from build123d import *

# Parameters (mm, degrees)
SKETCH1_W          = 120
SKETCH1_H          = 120
BASE_FLANGE1_DEPTH = 0.7366
EDGE_FLANGE1_DEPTH = 120
SKETCH25_R         = 1.5
CUT_EXTRUDE1_DEPTH = 161.891420775
CUT_EXTRUDE2_DEPTH = 10


# Sheet-metal steps are written as plain solids
with BuildPart() as part:
    # Sketch1 → Base-Flange1 (new body)
    with BuildSketch(Plane.XY):
        Rectangle(SKETCH1_W, SKETCH1_H)
    extrude(amount=-BASE_FLANGE1_DEPTH)

    # Edge-Flange1 section (across the edge) → Edge-Flange1 (add)
    with BuildSketch(Plane(origin=(-60, -61, 0), x_dir=(0, 1, 0), z_dir=(1, 0, 0))):
        with BuildLine():
            Line((-0.7366, 0.7366), (-0.7366, 24.2634))
            Line((-0.7366, 24.2634), (0, 24.2634))
            Line((0, 24.2634), (0, 0.7366))
            ThreePointArc((0, 0.7366), (0.215745145, 0.215745145), (0.7366, 0))
            Line((0.7366, 0), (1, 0))
            Line((1, 0), (1, -0.7366))
            Line((1, -0.7366), (0.7366, -0.7366))
            ThreePointArc((0.7366, -0.7366), (-0.30510971, -0.30510971), (-0.7366, 0.7366))
        make_face()
    extrude(amount=EDGE_FLANGE1_DEPTH)

    # Sketch25 → Cut-Extrude1 (cut, through all)
    with BuildSketch(Plane(origin=(-46.34767359, -57.645882303, 26.3866), x_dir=(1, 0, 0), z_dir=(0, 0, 1))):
        with Locations((-7.65232641, 6.745882303)):
            Circle(SKETCH25_R)
        with Locations((100.34767359, 113.545882303)):
            Circle(SKETCH25_R)
        with Locations((100.34767359, 6.745882303)):
            Circle(SKETCH25_R)
        with Locations((-7.65232641, 113.545882303)):
            Circle(SKETCH25_R)
    extrude(amount=-CUT_EXTRUDE1_DEPTH, mode=Mode.SUBTRACT)

    # Sketch26 → Cut-Extrude2 (cut)
    with BuildSketch(Plane(origin=(0, 0, -0.7366), x_dir=(-1, 0, 0), z_dir=(0, 0, -1))):
        Polygon((45, -15.899963077), (45, -0.320923852), (0.188671673, -45.2634), (15.722249294, -45.2634), align=None)
        Polygon((21.370855866, -45.2634), (36.904433487, -45.2634), (45, -37.144140463), (45, -21.565101238), align=None)
        Polygon((-20.993512521, -45.2634), (-5.459934899, -45.2634), (45, 5.344214309), (45, 20.923253534), align=None)
        Polygon((-45, -26.851791695), (-45, -42.43083092), (42.175696714, 45), (26.642119093, 45), align=None)
        Polygon((-45, -5.607614309), (-45, -21.186653534), (20.993512521, 45), (5.459934899, 45), align=None)
        Polygon((-45, 15.636563077), (-45, 0.057523852), (-0.188671673, 45), (-15.722249294, 45), align=None)
        Polygon((-45, 36.880740463), (-45, 21.301701238), (-21.370855866, 45), (-36.904433487, 45), align=None)
        Polygon((45, 26.588391695), (45, 42.16743092), (-42.175696714, -45.2634), (-26.642119093, -45.2634), align=None)
    extrude(amount=-CUT_EXTRUDE2_DEPTH, mode=Mode.SUBTRACT)


solid = part.part
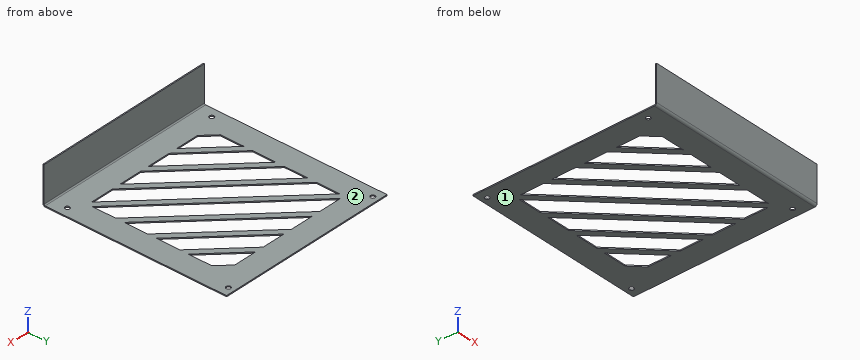
Could you check a few things on this model? Use its own coordinates, in mm. Face numbers are marked on the shaded views. A direction names the side the tool comes from. Coordinates: 2 decimals unless noted, no trailing zeros. Loops run counter-clockwise (first coordinate to the right, second up) from the corner with the lowest first, then second, coordinate; pieces in that order, holes last.
1. For P1, Ø6, axis at x = -11, y = -5.5, coming from the +Z side; P2, Ø6, axis at x = -22.5, z = 9, coming from the +Y side; P3, Ø0.8, axis at x = 4.5, z = -0.5, coming from the -Y side, each with a flat end and sliding along its axis, tell me the tip position at first contact or that it passes through.
2. Imagine slicing it at C-C (x = -23). Please give me the cut outline in (y, z).
3. Imagine slicing it at D-D (y = -11). Please give me the cut outline in (x, z), and give its area (3 significant figures).
4. Imagine slicing it at B-B (x = 54). Please give me the cut outline in (y, z), and give its area (3 significant figures).
5. Imagine slicing it at A-A (y = 55.9). Please give me the cut outline in (x, z).
6. For the marked faces 1 and 2, which set-ups out of +Z, -Z, +X, -X, +Y, -Y let a thin tool reach every point of the face, with its end or its side?
7. I need wall thicknesses on L1, parallel to Y at x = -54, z = -0.3; L2, parallel to Y at x = 54, z = -0.4; L3, parallel to Y at x = -19, z = 10.75. Which ranges of each line are inside material? Lowest first, please.
Computed values:
1. P1: stops at z = 0
1. P2: stops at y = -61
1. P3: stops at y = -61.48
2. outline: (-61.74, 0.74) arc R1.47 ccw to (-60.26, -0.74) - (-45.26, -0.74) - (-45.26, 0) - (-60.26, 0) arc R0.74 cw to (-61, 0.74) - (-61, 24.26) - (-61.74, 24.26) - close; (-43.63, -0.74) - (-37.96, -0.74) - (-37.96, 0) - (-43.63, 0) - close; (-22.39, -0.74) - (-16.72, -0.74) - (-16.72, 0) - (-22.39, 0) - close; (-1.14, -0.74) - (4.52, -0.74) - (4.52, 0) - (-1.14, 0) - close; (20.1, -0.74) - (25.77, -0.74) - (25.77, 0) - (20.1, 0) - close; (41.35, -0.74) - (60, -0.74) - (60, 0) - (41.35, 0) - close
3. outline: (-60, -0.74) - (-45, -0.74) - (-45, 0) - (-60, 0) - close; (-34.35, -0.74) - (-28.7, -0.74) - (-28.7, 0) - (-34.35, 0) - close; (-13.17, -0.74) - (-7.52, -0.74) - (-7.52, 0) - (-13.17, 0) - close; (8.01, -0.74) - (13.66, -0.74) - (13.66, 0) - (8.01, 0) - close; (29.19, -0.74) - (34.84, -0.74) - (34.84, 0) - (29.19, 0) - close; (45, -0.74) - (60, -0.74) - (60, 0) - (45, 0) - close
3. area: 38.7 mm2
4. outline: (-61.74, 0.74) arc R1.47 ccw to (-60.26, -0.74) - (-52.4, -0.74) - (-52.4, 0) - (-60.26, 0) arc R0.74 cw to (-61, 0.74) - (-61, 24.26) - (-61.74, 24.26) - close; (-49.4, -0.74) - (54.4, -0.74) - (54.4, 0) - (-49.4, 0) - close; (57.4, -0.74) - (60, -0.74) - (60, 0) - (57.4, 0) - close
4. area: 103 mm2
5. outline: (-60, -0.74) - (-55.5, -0.74) - (-55.5, 0) - (-60, 0) - close; (-52.5, -0.74) - (52.5, -0.74) - (52.5, 0) - (-52.5, 0) - close; (55.5, -0.74) - (60, -0.74) - (60, 0) - (55.5, 0) - close
6. face 1: -Z, +X, -X, +Y, -Y
6. face 2: +Z, +X, -X, +Y
7. L1: y = -61.31 to -52.4, -49.4 to 54.4, 57.4 to 60
7. L2: y = -61.2 to -52.4, -49.4 to 54.4, 57.4 to 60
7. L3: y = -61.74 to -61
